Work out the finished part from the listing and answer in its coordinate system (mm). Coordinates: 2 decimals unless noted, no trailing zeros. Loops run counter-clockwise (first coordinate to the right, second up) from the corner with the lowest first, then second, coordinate; pieces in that order, holes last. Notation, with made-up numbers: (27.25, 27.25) -> (50.25, 27.25) arc R13 cw to (50.25, 35.25) -> close; hole circle Ø2 at (-27, -30.5). An arc over 180 degrees is marked (long way). One line per question, with ' | ' between items.
Autodesk Inventor part; units mm, degrees
ref_plane "YZ Plane" through (0, 0, 0) normal (1, 0, 0) x (0, 1, 0)
ref_plane "XZ Plane" through (0, 0, 0) normal (0, 1, 0) x (-1, 0, 0)
ref_plane "XY Plane" through (0, 0, 0) normal (0, 0, 1) x (1, 0, 0)
sketch "Эскиз1" plane through (0, 0, 0) normal (0, 1, 0) x (-1, 0, 0)
  line L0 (-275, 275) -> (275, 275)
  line L1 (275, 275) -> (275, -275)
  line L2 (275, -275) -> (-275, -275)
  line L3 (-275, -275) -> (-275, 275)
  line L4 (-275, 275) -> (275, -275) construction
  line L5 (275, 275) -> (-275, -275) construction
  circle A0 centre (200, -200) radius 10.5
  circle A1 centre (200, 0) radius 10.5
  circle A2 centre (200, 200) radius 10.5
  circle A3 centre (0, 200) radius 10.5
  circle A4 centre (-200, 200) radius 10.5
  circle A5 centre (-200, 0) radius 10.5
  circle A6 centre (-200, -200) radius 10.5
  circle A7 centre (0, -200) radius 10.5
  circle A8 centre (0, 0) radius 137.5 construction
  circle A9 centre (0, -137.5) radius 8.5
  circle A10 centre (97.2272, -97.2272) radius 8.5
  circle A11 centre (137.5, 0) radius 8.5
  circle A12 centre (97.2272, 97.2272) radius 8.5
  circle A13 centre (0, 137.5) radius 8.5
  circle A14 centre (-97.2272, 97.2272) radius 8.5
  circle A15 centre (-137.5, 0) radius 8.5
  circle A16 centre (-97.2272, -97.2272) radius 8.5
  dimension "d7" = 275
  dimension "d0" = 550
  dimension "d1" = 550
  dimension "d2" = 75
  dimension "d3" = 75
  dimension "d4" = 75
  dimension "d5" = 75
  dimension "d6" = 21
  dimension "d8" = 17
  dimension "d11" = 360
extrude "Пластина1" add sketch "Эскиз1" along normal blind 20
equation "\"d13\" = Толщина"
properties part number "Lift.02.00.00.06" material "Сталь нержавеющая, 440C"
1) Find the intervals of material crossed by line 1 along Z through (x, y) = (0, 11.5); line 2 along Z through (x, y) = (-200, 12); line 3 along Z through (x, y) = (137.5, 12.5), in increasing order.
Check values:
line 1: z = -275 to -210.5, -189.5 to -146, -129 to 129, 146 to 189.5, 210.5 to 275 | line 2: z = -275 to -210.5, -189.5 to -10.5, 10.5 to 189.5, 210.5 to 275 | line 3: z = -275 to -8.5, 8.5 to 275
2) The mould has two halves that part along Z. Classify faces 1 (the face through (-95.385, 9.86, 105.525)), 2 (the face through (4, 20, 4)): released by +Z, released by -Z, zero draft, split by the parting line, or undercut.
Check values:
face 1: undercut | face 2: zero draft
3) Find section B-B (z = 137.5). Write down the section's boundary in (x, y), plus the area to 3 significant figures.
Check values:
outline: (-275, 0) -> (-8.5, 0) -> (-8.5, 20) -> (-275, 20) -> close; (8.5, 0) -> (275, 0) -> (275, 20) -> (8.5, 20) -> close | area: 10,700 mm^2
4) Find section C-C (z = 200). Write down the section's boundary in (x, y), plus the area to 3 significant figures.
Check values:
outline: (-275, 0) -> (-210.5, 0) -> (-210.5, 20) -> (-275, 20) -> close; (-189.5, 0) -> (-10.5, 0) -> (-10.5, 20) -> (-189.5, 20) -> close; (10.5, 0) -> (189.5, 0) -> (189.5, 20) -> (10.5, 20) -> close; (210.5, 0) -> (275, 0) -> (275, 20) -> (210.5, 20) -> close | area: 9,740 mm^2
5) Find section A-A (x = -200). Write down the section's boundary in (y, z).
Check values:
outline: (0, -275) -> (20, -275) -> (20, -210.5) -> (0, -210.5) -> close; (0, -189.5) -> (20, -189.5) -> (20, -10.5) -> (0, -10.5) -> close; (0, 10.5) -> (20, 10.5) -> (20, 189.5) -> (0, 189.5) -> close; (0, 210.5) -> (20, 210.5) -> (20, 275) -> (0, 275) -> close
6) Find section D-D (x = -137.5). Write down the section's boundary in (y, z), plus the area to 3 significant figures.
Check values:
outline: (0, -275) -> (20, -275) -> (20, -8.5) -> (0, -8.5) -> close; (0, 8.5) -> (20, 8.5) -> (20, 275) -> (0, 275) -> close | area: 10,700 mm^2
7) A flat-ended cylindrical pin translates along its axis: pin 1 (22 mm diameter, centred on x = 97.23, z = -97.23, fed in from +Y). Find the tip coordinate at first contact, or state that the pin passes through.
Check values:
pin 1: stops at y = 20
